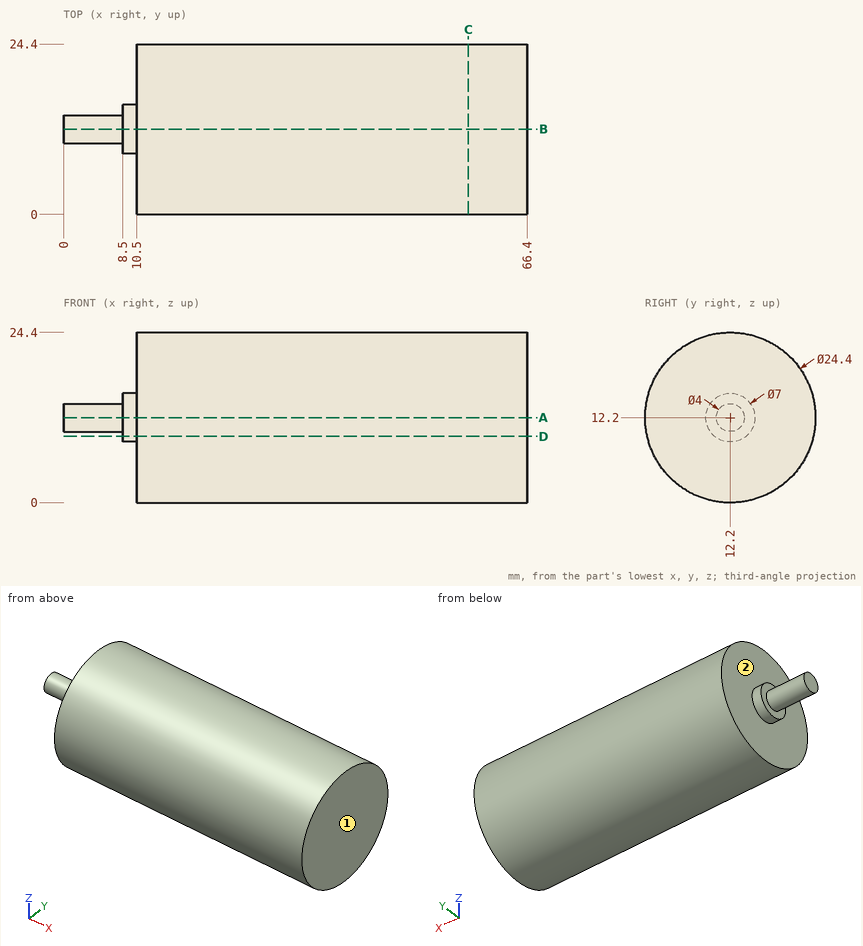
Can you work these out from the drawing? Everything is in mm from the part's minimum corner. A direction names the side the tool comes from. Give positions to 0.01 mm unless a question says otherwise; leave off trailing zeros. Order: outer loops, then holes, each group sorted by start corner. A loop starts at its lowest first (then second) coordinate and runs counter-clockwise, first axis right, second up.
Item 1: For the marked faces 1 and 2, which set-ups out of +Z, -Z, +X, -X, +Y, -Y let a thin tool reach every point of the face, with its end or its side?
Item 2: I need wall thicknesses on line 1 (X direction, y = 22.25, z = 6.5); line 2 (Y direction, x = 23, z = 19.75); line 3 (Y direction, x = 7, z = 12.25). Which ranges of each line are inside material? Lowest first, please.
Item 3: I'm going to push flat-ended pins straight in: pin 1 (8 mm diameter, centred on y = 20.5, z = 14, fed in from -X); pin 2 (4 mm diameter, centred on x = 10.5, z = 13.5, fed in from +Y); pin 3 (2 mm diameter, centred on x = 58.5, z = 5.5, fed in from +Y); pin 4 (10 mm diameter, centred on x = 58.5, y = 21.5, fed in from +Z). Where does each tip first touch, or does it pass through?
Item 4: If we section it at D-D, the plane z = 9.5: Write out the boundary of the cut face in (x, y).
Item 5: If we section it at A-A, the plane z = 12.2: Write out the boundary of the cut face in (x, y).
Item 6: If we section it at C-C, the plane x = 58: Write out the boundary of the cut face in (y, z).
Values:
1. face 1: +Z, -Z, +X, +Y, -Y
1. face 2: -X
2. line 1: x = 10.5 to 66.4
2. line 2: y = 2.62 to 21.78
2. line 3: y = 10.2 to 14.2
3. pin 1: stops at x = 10.5
3. pin 2: stops at y = 24.4
3. pin 3: stops at y = 22.99
3. pin 4: stops at z = 23.62
4. outline: (8.5, 9.97) - (10.5, 9.97) - (10.5, 0.3) - (66.4, 0.3) - (66.4, 24.1) - (10.5, 24.1) - (10.5, 14.43) - (8.5, 14.43) - close
5. outline: (0, 10.2) - (8.5, 10.2) - (8.5, 8.7) - (10.5, 8.7) - (10.5, 0) - (66.4, 0) - (66.4, 24.4) - (10.5, 24.4) - (10.5, 15.7) - (8.5, 15.7) - (8.5, 14.2) - (0, 14.2) - close
6. outline: circle Ø24.4 at (12.2, 12.2)
